CAD build for the part. Positions are in the model's coordinates, mm. A direction names the side the tool comes from. Round coordinates to 2 decimals unless told otherwise and drop trailing zeros. Order: outer loops, then holes, each group sorted by start corner. A loop starts at its lowest first (then second) coordinate and runs counter-clockwise, first axis right, second up. Notation, with made-up numbers: (25.5, -38) -> (40.5, -38) arc R20 cw to (40.5, -18) -> close; hole circle Ø4 at (74.5, 79). An arc over 180 degrees is marked (long way). Answer as CSV lines item,"result". Start each with the question number.
from build123d import *

# Parameters (mm, degrees)
SKETCH1_W           = 13
SKETCH1_H           = 15
BOSS_EXTRUDE1_DEPTH = 19
SKETCH2_R           = 1.57
BOSS_EXTRUDE2_DEPTH = 4.75
SKETCH3_R           = 1.5
BOSS_EXTRUDE3_DEPTH = 5.5
CUT_EXTRUDE1_DEPTH  = 0.5
CUT_EXTRUDE2_DEPTH  = 0.5


with BuildPart() as part:
    # Sketch1 → Boss-Extrude1 (new body)
    with BuildSketch(Plane.XY):
        Rectangle(SKETCH1_W, SKETCH1_H)
    extrude(amount=BOSS_EXTRUDE1_DEPTH)

    # Sketch2 → Boss-Extrude2 (add)
    with BuildSketch(Plane.XY.offset(19)):
        Circle(SKETCH2_R)
    extrude(amount=BOSS_EXTRUDE2_DEPTH)

    # Sketch3 → Boss-Extrude3 (add)
    with BuildSketch(Plane(origin=(0, 0, 0), x_dir=(-1, 0, 0), z_dir=(0, 0, -1))):
        Circle(SKETCH3_R)
    extrude(amount=BOSS_EXTRUDE3_DEPTH)

    # Sketch4 → Cut-Extrude1 (cut)
    with BuildSketch(Plane(origin=(0, 0, 0), x_dir=(-1, 0, 0), z_dir=(0, 0, -1))):
        Polygon((-2.028652102, -5.782501305), (-1.56661284, -2.282501305), (-1.521741045, -2.282501305), (-0.076729025, -5.154296177), (1.364076263, -2.282501305), (1.408948058, -2.282501305), (1.875194051, -5.782501305), (1.561091487, -5.782501305), (1.224553026, -3.266175183), (-0.038167327, -5.782501305), (-0.10968175, -5.782501305), (-1.378011077, -3.258462844), (-1.712446173, -5.782501305), align=None)
    extrude(amount=-CUT_EXTRUDE1_DEPTH, mode=Mode.SUBTRACT)

    # Sketch5 → Cut-Extrude2 (cut)
    with BuildSketch(Plane.XY.offset(19)):
        with BuildLine():
            Line((-0.851399992, -2.584854315), (-0.165001755, -2.584854315))
            add(Edge.make_bspline(
                [(-0.165001755, -2.584854315), (-0.117790848, -2.584906211), (-0.027332656, -2.585005646), (0.1023824, -2.588020392), (0.220192132, -2.592047084), (0.325842513, -2.597628978), (0.419658611, -2.604225568), (0.50121591, -2.613477607), (0.571155467, -2.623137903), (0.613061916, -2.632959309), (0.632173726, -2.637438449)],
                knots=[0, 0, 0, 0, 0.000141628, 0.000271366, 0.00038923, 0.000495248, 0.00058876, 0.000671296, 0.000741499, 0.00080036, 0.00080036, 0.00080036, 0.00080036], degree=3))
            add(Edge.make_bspline(
                [(0.632173726, -2.637438449), (0.65636726, -2.644060399), (0.704184237, -2.657148261), (0.77308528, -2.683361984), (0.838639126, -2.71444415), (0.901070684, -2.749868089), (0.959612767, -2.791153654), (1.015138808, -2.836627271), (1.067158788, -2.88733884), (1.11538018, -2.94271958), (1.159664978, -3.00183979), (1.197794661, -3.06558202), (1.229721888, -3.132873323), (1.257105159, -3.203666894), (1.276813614, -3.278557218), (1.291660513, -3.35702393), (1.301084141, -3.43905862), (1.301986703, -3.495118488), (1.302446162, -3.523656398)],
                knots=[0, 0, 0, 0, 7.5216e-05, 0.00014866, 0.000220794, 0.000292713, 0.000363707, 0.000435434, 0.000507823, 0.000581364, 0.000655543, 0.000729131, 0.000803767, 0.000878771, 0.000956497, 0.001035702, 0.001118238, 0.001203821, 0.001203821, 0.001203821, 0.001203821], degree=3))
            add(Edge.make_bspline(
                [(1.302446162, -3.523656398), (1.302024737, -3.552434175), (1.301200191, -3.608739839), (1.291303906, -3.691112627), (1.277973714, -3.769831017), (1.257476662, -3.844720468), (1.230630989, -3.915336238), (1.199138936, -3.98275747), (1.161155406, -4.045837142), (1.117510576, -4.10480426), (1.068958982, -4.159714172), (1.015706044, -4.210168966), (0.957966751, -4.255873305), (0.895924603, -4.296929648), (0.828974754, -4.332385928), (0.758132601, -4.364143233), (0.682782384, -4.390814293), (0.63063987, -4.404844355), (0.604128854, -4.411977712)],
                knots=[0, 0, 0, 0, 8.6284e-05, 0.00016882, 0.000248587, 0.000325638, 0.000401297, 0.000474998, 0.000548586, 0.000621785, 0.0006948, 0.0007682, 0.000841564, 0.000915458, 0.000991056, 0.00106858, 0.00114819, 0.001230532, 0.001230532, 0.001230532, 0.001230532], degree=3))
            add(Edge.make_bspline(
                [(0.604128854, -4.411977712), (0.58220152, -4.416640693), (0.534146493, -4.426859887), (0.455003771, -4.438268344), (0.362858385, -4.448005945), (0.257836105, -4.455307082), (0.1400312, -4.461557451), (0.009379943, -4.466525545), (-0.134374134, -4.469255399), (-0.234645379, -4.469396191), (-0.286996947, -4.469469699)],
                knots=[0, 0, 0, 0, 6.7238e-05, 0.000147357, 0.000239727, 0.000345177, 0.000463135, 0.000593636, 0.000737393, 0.000894446, 0.000894446, 0.000894446, 0.000894446], degree=3))
            Line((-0.286996947, -4.469469699), (-0.537297428, -4.469469699))
            Line((-0.537297428, -4.469469699), (-0.537297428, -6.084854315))
            Line((-0.537297428, -6.084854315), (-0.851399992, -6.084854315))
            Line((-0.851399992, -6.084854315), (-0.851399992, -2.584854315))
        make_face()
        with BuildLine():
            Line((-0.537297428, -2.943828674), (-0.537297428, -4.11049534))
            Line((-0.537297428, -4.11049534), (0.075483021, -4.11820768))
            add(Edge.make_bspline(
                [(0.075483021, -4.11820768), (0.105402947, -4.118223144), (0.163162747, -4.118252996), (0.24659897, -4.114267772), (0.324008257, -4.10966724), (0.395152833, -4.102931316), (0.460064767, -4.093410059), (0.518852296, -4.083798321), (0.571059579, -4.069892958), (0.632158781, -4.051169889), (0.700242128, -4.019237273), (0.774309677, -3.972887383), (0.837080263, -3.913806675), (0.89139856, -3.847378844), (0.934504438, -3.773479714), (0.96606043, -3.694410778), (0.984601587, -3.610982928), (0.987087781, -3.553894789), (0.988343598, -3.525058642)],
                knots=[0, 0, 0, 0, 8.9746e-05, 0.000173253, 0.000250533, 0.00032239, 0.000387534, 0.00044736, 0.000500926, 0.000549486, 0.000638903, 0.000725641, 0.000810488, 0.000896226, 0.000982324, 0.00106604, 0.001150757, 0.001237226, 0.001237226, 0.001237226, 0.001237226], degree=3))
            add(Edge.make_bspline(
                [(0.988343598, -3.525058642), (0.987080951, -3.496920128), (0.984570966, -3.440984246), (0.965915103, -3.359005485), (0.934565789, -3.280769781), (0.891109195, -3.207796696), (0.838368065, -3.141607892), (0.777068722, -3.084110765), (0.707355461, -3.037889062), (0.642507229, -3.00805578), (0.584906043, -2.989840505), (0.534874084, -2.977095664), (0.478383409, -2.966920058), (0.41541563, -2.958680555), (0.346458796, -2.951627094), (0.270920481, -2.946841117), (0.189086838, -2.944039661), (0.132276267, -2.943900705), (0.102826771, -2.943828674)],
                knots=[0, 0, 0, 0, 8.4371e-05, 0.000167719, 0.000250783, 0.000336277, 0.000421575, 0.000503926, 0.000587348, 0.000671427, 0.000717102, 0.000768457, 0.000826213, 0.000889178, 0.000958942, 0.001034123, 0.001116202, 0.001204546, 0.001204546, 0.001204546, 0.001204546], degree=3))
            Line((0.102826771, -2.943828674), (-0.537297428, -2.943828674))
        make_face(mode=Mode.SUBTRACT)
    extrude(amount=-CUT_EXTRUDE2_DEPTH, mode=Mode.SUBTRACT)


solid = part.part
Item 1: Band-saw the part on B-B, the plane x = -3.5. Give the cut face in (y, z).
Item 2: Mould opens along Y. For faces 5 (the cylindrical face through (1.5, 0.07, -2.71)), 6 (the flat face through (0.81, -3.7, 0.25)), 7 (the flat face through (0, 7.5, 9)), 8 (the flat face through (-2, 0, 0)) say: released by +Y, released by -Y, zero draft, split by the parting line, or undercut.
Item 3: Pin check, flat tips, straight feed: pin 1 (2.5 mm diameter, centred on x = 0.5, y = -4, fed in from +Z); pin 2 (1 mm diameter, centred on x = 4, y = -4.5, fed in from -Z). Stop position of each tip, or through.
Item 4: Band-saw the part on C-C, the plane z = -1.75. Give the cut face in (x, y).
Item 5: Tool access for faces 1 (the flat face through (-0.6, -4.51, 0.25)), 2 (the cylindrical face through (1.5, 0.47, 21.34)), 3 (the flat face through (0, 0, -5.5)), 4 (the flat face through (0.2, -3.5, 19)): list every direction of +Z, -Z, +X, -X, +Y, -Y with a clear straight run to the whole face (end or side of a thin tool).
Item 6: Probe line 1 (Z direction, x = -5, y = -6.5); line 2 (Z direction, x = 0.5, y = -4.75); line 3 (X direction, y = 0.5, z = 19.5). List the from-to ranges inside material, lowest first.
Item 7: Band-saw the part on A-A, the plane y = 0. Give the cut face in (x, z), and give its area (3 significant figures).
Item 8: Band-saw the part on D-D, the plane y = 5.5. Give the cut face in (x, z), and give its area (3 significant figures).
Values:
1,outline,"(-7.5, 0) -> (7.5, 0) -> (7.5, 19) -> (-7.5, 19) -> close"
2,face 5,"split by the parting line"
2,face 6,"undercut"
2,face 7,"released by +Y"
2,face 8,"zero draft"
3,pin 1,"z = 19"
3,pin 2,"z = 0"
4,outline,"circle Ø3 at (0, 0)"
5,face 1,"-Z"
5,face 2,"+Z"
5,face 3,"-Z, +X, -X, +Y, -Y"
5,face 4,"+Z, +X, -X, -Y"
6,line 1,"0 to 19"
6,line 2,"0.5 to 19"
6,line 3,"-1.49 to 1.49"
7,outline,"(-6.5, 0) -> (-1.5, 0) -> (-1.5, -5.5) -> (1.5, -5.5) -> (1.5, 0) -> (6.5, 0) -> (6.5, 19) -> (1.57, 19) -> (1.57, 23.75) -> (-1.57, 23.75) -> (-1.57, 19) -> (-6.5, 19) -> close"
7,area,"278 mm²"
8,outline,"(-6.5, 0) -> (6.5, 0) -> (6.5, 19) -> (-6.5, 19) -> close"
8,area,"247 mm²"
